Design review of the part built by this model. Coordinates are the model's own, in mm. A direction names the side the tool comes from. Coordinates: 2 decimals unless noted, no trailing zeros. Order: outer loops, then holes, each group sorted by start corner. A loop starts at its lowest first (then second) coordinate and runs counter-clockwise, first axis right, second up. Notation, with made-up numbers: (81.25, 5) - (111.25, 5) arc R21 cw to (111.25, 17) - close; hole circle Ø10 at (53, -7). An arc over 180 degrees is marked (long way). Write each question's results on one line, items separated by ' | '. Start each with the question number.
```python
from build123d import *

# Parameters (mm, degrees)
SKETCH_1_W          = 42.3
SKETCH_1_H          = 42.3
EXTRUDE_1_DEPTH     = 34.5
SKETCH_2_R          = 11
EXTRUDE_2_DEPTH     = 2
SKETCH_3_R          = 1.5
CUT_EXTRUDE_1_DEPTH = 5
SKETCH_4_R          = 4
CUT_EXTRUDE_2_DEPTH = 37.5
CHAMFER_1_SIZE      = 4


with BuildPart() as part:
    # 草图1 → 凸台-拉伸1 (new body)
    with BuildSketch(Plane(origin=(0, 0, 0), x_dir=(1, 0, 0), z_dir=(0, 1, 0))):
        Rectangle(SKETCH_1_W, SKETCH_1_H)
    extrude(amount=EXTRUDE_1_DEPTH)

    # 草图2 → 凸台-拉伸2 (add)
    with BuildSketch(Plane(origin=(0, 34.5, 0), x_dir=(1, 0, 0), z_dir=(0, 1, 0))):
        Circle(SKETCH_2_R)
    extrude(amount=EXTRUDE_2_DEPTH)

    # 草图3 → 切除-拉伸1 (cut)
    with BuildSketch(Plane(origin=(0, 34.5, 0), x_dir=(1, 0, 0), z_dir=(0, 1, 0))):
        with Locations((-15.5, 15.5)):
            Circle(SKETCH_3_R)
        with Locations((15.5, 15.5)):
            Circle(SKETCH_3_R)
        with Locations((15.5, -15.5)):
            Circle(SKETCH_3_R)
        with Locations((-15.5, -15.5)):
            Circle(SKETCH_3_R)
    extrude(amount=-CUT_EXTRUDE_1_DEPTH, mode=Mode.SUBTRACT)

    # 草图4 → 切除-拉伸2 (cut, through all)
    with BuildSketch(Plane(origin=(0, 36.5, 0), x_dir=(1, 0, 0), z_dir=(0, 1, 0))):
        Circle(SKETCH_4_R)
    extrude(amount=-CUT_EXTRUDE_2_DEPTH, mode=Mode.SUBTRACT)

    # 倒角1
    chamfer_1_edges = [part.edges().sort_by_distance(p)[0] for p in [
        (21.15, 17.25, 21.15),
        (-21.15, 17.25, 21.15),
        (-21.15, 17.25, -21.15),
        (21.15, 17.25, -21.15),
    ]]
    chamfer(chamfer_1_edges, length=CHAMFER_1_SIZE)


solid = part.part
```
(1) Take a section at C-C (y = 12). State the section outline as (x, z) points.
(2) To check wall thickness, follow line 1 along Z through (x, y) = (15.5, 31.15); line 2 along X through (y, z) = (29, 0). State the ranges of each line that lie inside material, in increasing order. Write a range as [from, to].
(3) Mouldability with a two-part tool opening along X and no side actions: class faces 1 (the face through (0, 36.5, 5)), 2 (the face through (-0.867, 18.506, 3.905)), 3 (the face through (-16, 29.5, -16)), 4 (the face through (-19.1, 17, -19.2)) as +X half, -X half, draft (parallel to the pull), parting line (faces both ways), or undercut.
(4) Take a section at B-B (x = 0). State the section outline as (y, z) points.
(5) Take a section at A-A (z = 0). State the section outline as (x, y) points.
(6) Take a section at D-D (x = 15.5). State the section outline as (y, z) points, plus the area to 3 significant figures.
(7) Tool access review of faces 5 (the face through (0, 17, 21.15)), 6 (the face through (15, 29.5, 15)): name each direction out of +Z, -Z, +X, -X, +Y, -Y from which nothing blocks a thin tool from reaching the whole face with its end or side.
(8) Clearance check with flat-ended pins moving along their axes: pin 1 (0.9 mm diameter, centred on x = 15.5, z = 15.5, fed in from +Y); pin 2 (3.5 mm diameter, centred on x = -15.5, z = 15.5, fed in from +Y). State where each tip first meets the part, or that it passes through.
Worked out:
1) outline: (-21.15, -17.15) - (-17.15, -21.15) - (17.15, -21.15) - (21.15, -17.15) - (21.15, 17.15) - (17.15, 21.15) - (-17.15, 21.15) - (-21.15, 17.15) - close; hole circle Ø8 at (0, 0)
2) line 1: [-21.15, -17], [-14, 14], [17, 21.15] | line 2: [-21.15, -4], [4, 21.15]
3) face 1: draft | face 2: undercut | face 3: undercut | face 4: -X half
4) outline: (0, -21.15) - (34.5, -21.15) - (34.5, -11) - (36.5, -11) - (36.5, -4) - (0, -4) - close; (0, 4) - (36.5, 4) - (36.5, 11) - (34.5, 11) - (34.5, 21.15) - (0, 21.15) - close
5) outline: (-21.15, 0) - (-4, 0) - (-4, 36.5) - (-11, 36.5) - (-11, 34.5) - (-21.15, 34.5) - close; (4, 0) - (21.15, 0) - (21.15, 34.5) - (11, 34.5) - (11, 36.5) - (4, 36.5) - close
6) outline: (0, -21.15) - (34.5, -21.15) - (34.5, -17) - (29.5, -17) - (29.5, -14) - (34.5, -14) - (34.5, 14) - (29.5, 14) - (29.5, 17) - (34.5, 17) - (34.5, 21.15) - (0, 21.15) - close | area: 1,430 mm^2
7) face 5: +Z, +X, -X, +Y, -Y | face 6: +Y
8) pin 1: y = 29.5 | pin 2: y = 34.5
